from build123d import *

# Parameters (mm, degrees)
F1_DEPTH = 15


with BuildPart() as f1:
    # F0 (on Front) → F1 (new body)
    with BuildSketch(Plane.XZ):
        with BuildLine():
            Line((-50.211565, 7.379583), (-49.536289, 6.907117))
            ThreePointArc((-49.536289, 6.907117), (-48.215818, -8.066107), (-33.540352, -4.814682))
            Line((-33.540352, -4.814682), (-32.444857, -5.16249))
            ThreePointArc((-32.444857, -5.16249), (-31.720531, -5.116098), (-31.218368, -4.592044))
            ThreePointArc((-31.218368, -4.592044), (-30.591796, 2.607902), (-34.213844, 8.861907))
            Line((-34.213844, 8.861907), (-30.920298, 12.905683))
            ThreePointArc((-30.920298, 12.905683), (-30.167371, 13.273918), (-29.398681, 12.939833))
            Line((-29.398681, 12.939833), (-16.410195, -1.621093))
            Line((-16.410195, -1.621093), (-7.871556, -1.621093))
            Line((-7.871556, -1.621093), (-0.642441, 0.20388))
            ThreePointArc((-0.642441, 0.20388), (0.188985, 0.044133), (0.599902, -0.696093))
            ThreePointArc((0.599902, -0.696093), (18.599287, -5.968348), (8.373546, 9.754525))
            ThreePointArc((8.373546, 9.754525), (7.359995, 9.987757), (6.909294, 10.925068))
            Line((6.909294, 10.925068), (6.909294, 11.237489))
            ThreePointArc((6.909294, 11.237489), (7.180434, 11.922151), (7.846819, 12.235535))
            Line((7.846819, 12.235535), (21.346842, 13.080605))
            ThreePointArc((21.346842, 13.080605), (21.933025, 13.597725), (21.577048, 14.293644))
            Line((21.577048, 14.293644), (11.140821, 19.176345))
            ThreePointArc((11.140821, 19.176345), (10.877845, 19.236347), (10.613608, 19.182167))
            Line((10.613608, 19.182167), (0, 14.499336))
            Line((0, 14.499336), (-7.632633, 14.499336))
            Line((-7.632633, 14.499336), (-15.239003, 18.976845))
            Line((-15.239003, 18.976845), (-29.227387, 20.273161))
            Line((-29.227387, 20.273161), (-26.190706, 24.307124))
            Line((-26.190706, 24.307124), (-22.441075, 22.722935))
            ThreePointArc((-22.441075, 22.722935), (-21.077169, 22.823507), (-20.361762, 23.989073))
            Line((-20.361762, 23.989073), (-20.355286, 24.072853))
            ThreePointArc((-20.355286, 24.072853), (-20.498198, 24.670009), (-20.963128, 25.071082))
            Line((-20.963128, 25.071082), (-24.808915, 26.695896))
            ThreePointArc((-24.808915, 26.695896), (-26.070014, 26.794443), (-27.13801, 26.116602))
            Line((-27.13801, 26.116602), (-39.011024, 11.539056))
            ThreePointArc((-39.011024, 11.539056), (-44.991956, 11.695307), (-50.304952, 8.944303))
            ThreePointArc((-50.304952, 8.944303), (-50.636512, 8.139368), (-50.211565, 7.379583))
        make_face()
    extrude(amount=F1_DEPTH)


solid = f1.part
Check sheet for the modelled part. Datum: model origin and axes. Units: mm. A direction names the side the tool comes from. Round coordinates to 2 decimals unless told otherwise and drop trailing zeros. Loops run counter-clockwise (first coordinate to the right, second up) from the corner with the lowest first, then second, coordinate; pieces in that order, holes last.
1. Sectioned sample at A-A on z = 1. Record the boundary of the cut face in (x, y).
2. Scan lines: probe 1 along X at (y, z) = (-6.5, 5); probe 2 along X at (y, z) = (-8.5, 1.5); probe 3 along Z at (x, y) = (-29, -13.5). Record each from-to range of solid material in increasing order.
3. Mould release check, pull along Z, two halves, no side actions. Record for faces 1 (the cylindrical face through (7.37, -7.4, 9.98)), 2 (the flat face through (-12, -7, -1.621)), 3 (the flat face through (16.43, -7.4, 16.7)), 4 (the flat face through (-16, 0, 5)): released by +Z, released by -Z, zero draft, split by the parting line, or undercut.
4. Sectioned sample at B-B on x = -23.5. Record the boundary of the cut face in (y, z).
5. Gauge pin test, flat ends, axial feed: pin 1 Ø5 at (x, y) = (-0.5, -11.5) entering from +Z; pin 2 Ø5 at (x, y) = (-44, -11.5) entering from -Z; pin 3 Ø4 at (x, y) = (-5, -6.5) entering from +Z; pin 4 Ø7 at (x, y) = (-11.5, -4) entering from -Z. Record the tip position at first contact, or that the pin passes through.
6. Set-up check for faces 5 (the flat face through (-16, -15, 5)), 6 (the flat face through (-27.7, -7.4, 22.3)), 7 (the flat face through (5.381, -7.395, 16.874)), 8 (the flat face through (-22.995, -7.395, 5.761)): record each of +Z, -Z, +X, -X, +Y, -Y from which the full face is reachable in a straight line by a thin tool's end or side.
Recorded:
1. outline: (-52.25, -15) - (-30.35, -15) - (-30.35, 0) - (-52.25, 0) - close; (-18.75, -15) - (20.53, -15) - (20.53, 0) - (-18.75, 0) - close
2. probe 1: x = -50.97 to -31.4, -22.32 to 19.24
2. probe 2: x = -52.19 to -30.4, -19.19 to 20.46
2. probe 3: z = 12.49 to 20.25, 20.58 to 23.83
3. face 1: undercut
3. face 2: released by -Z
3. face 3: released by +Z
3. face 4: zero draft
4. outline: (-15, 6.33) - (0, 6.33) - (0, 19.74) - (-15, 19.74) - close; (-15, 23.17) - (0, 23.17) - (0, 26.14) - (-15, 26.14) - close
5. pin 1: stops at z = 15.38
5. pin 2: stops at z = -10
5. pin 3: stops at z = 14.5
5. pin 4: stops at z = -1.62
6. face 5: +Z, -Z, +X, -X, -Y
6. face 6: +Y, -Y
6. face 7: +Z, +Y, -Y
6. face 8: -Z, +Y, -Y
